Can you work these out from the model? Positions are in its coordinate system, mm. Face numbers are marked on the shaded views. A direction names the side the tool comes from. Give positions to 0.01 mm unless a question says otherwise; leave off trailing zeros. Order: outer loops, then holes, each group sorted by start corner. A loop starts at its lowest first (then second) coordinate and runs counter-clockwise, first axis right, second up. Notation, with made-up numbers: (29.25, 36.25) -> (46.25, 36.25) arc R25 cw to (46.25, 71.25) -> close; hole circle Ø11 at (51, -29.5). An arc over 180 degrees is marked (long way). Answer as a JSON object with one key per item and string values.
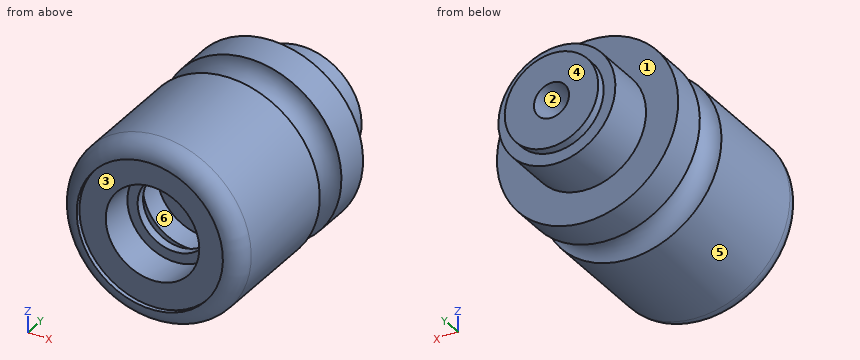
```python
from build123d import *

# Parameters (mm, degrees)
F0_W     = 30
F0_H     = 160
F2_W     = 30
F2_H     = 125
F2_W_2   = 80
F2_H_2   = 160
F4_R     = 60
F5_DEPTH = 580.001


with BuildPart() as f1:
    # F0 (on Right) → F1 (revolve)
    with BuildSketch(Plane.YZ):
        with BuildLine():
            Line((0, 250), (0, 0))
            Line((0, 0), (680, 0))
            Line((680, 0), (680, 200))
            Line((680, 200), (680, 310))
            Line((680, 310), (560, 310))
            ThreePointArc((560, 310), (500, 250), (440, 310))
            Line((440, 310), (60, 310))
            ThreePointArc((60, 310), (17.573593, 292.426407), (0, 250))
        make_face()
        Polygon((680, 200), (680, 0), (850, 0), (850, 160), (850, 200), align=None)
        with Locations((865, 80)):
            Rectangle(F0_W, F0_H)
    revolve(axis=Axis((0, 440, 0), (0, 1, 0)))

    # F2 (on Right) → F3 (revolve, cut)
    with BuildSketch(Plane.YZ):
        Polygon((0, 250), (0, 0), (15, 0), (15, 160), (15, 250), align=None)
        Polygon((15, 160), (15, 0), (135, 0), (135, 125), (135, 160), align=None)
        with Locations((150, 62.5)):
            Rectangle(F2_W, F2_H)
        Polygon((165, 125), (165, 0), (220, 0), (220, 160), (220, 205), (165, 205), align=None)
        with Locations((260, 80)):
            Rectangle(F2_W_2, F2_H_2)
    revolve(axis=Axis((0, 192.5, 0), (0, 1, 0)), mode=Mode.SUBTRACT)

    # F4 (on face) → F5 (cut, through all)
    with BuildSketch(Plane.XZ.offset(-300)):
        Circle(F4_R)
    extrude(amount=-F5_DEPTH, mode=Mode.SUBTRACT)


solid = f1.part
```
1. For the marked faces 1, 2 and 3, which set-ups out of +Z, -Z, +X, -X, +Y, -Y let a thin tool reach every point of the face, with its end or its side?
Worked answers:
{"face 1": "+Y", "face 2": "+Y, -Y", "face 3": "-Y"}
2. If we mould it in two halves opening along Z, with no side actions, what happens to the marked faces 4, 5 and 6? For each: +Z half, -Z half, draft (parallel to the pull), parting line (faces both ways), or undercut.
Worked answers:
{"face 4": "draft", "face 5": "parting line", "face 6": "undercut"}
3. If we section it at A-A on y = 722.5: Please give me the cut outline in (x, z).
Worked answers:
{"outline": "circle Ø400 at (0, 0); hole circle Ø120 at (0, 0)"}
4. Please list where these lines run through material, in increasing order: L1, parallel to X at y = 190.5, z = 0; L2, parallel to X at y = 152.5, z = 0; L3, parallel to Y at x = 108, z = 147.5.
Worked answers:
{"L1": "-310 to -205, 205 to 310", "L2": "-310 to -125, 125 to 310", "L3": "15 to 165, 220 to 850"}
5. Will these pins go through, and if not, where does the flat tip stop? pin 1 Ø10 at (x, z) = (-163.5, -21.5) entering from -Y; pin 2 Ø10 at (x, y) = (-79, 722) entering from +Z; pin 3 Ø1.5 at (x, y) = (-139, 375) entering from -Z.
Worked answers:
{"pin 1": "y = 15", "pin 2": "z = 185.81", "pin 3": "z = -277.47"}
